from build123d import *

# Parameters (mm, degrees)
SKETCH1_R           = 8.5
SKETCH1_R_2         = 4.5
BOSS_EXTRUDE1_DEPTH = 2.5
SKETCH2_R           = 8
SKETCH2_R_2         = 5
CUT_EXTRUDE1_DEPTH  = 0.1


with BuildPart() as part:
    # Sketch1 → Boss-Extrude1 (new body, symmetric)
    with BuildSketch(Plane(origin=(0, 0, 0), x_dir=(1, 0, 0), z_dir=(0, 1, 0))):
        Circle(SKETCH1_R)
        Circle(SKETCH1_R_2, mode=Mode.SUBTRACT)
    extrude(amount=BOSS_EXTRUDE1_DEPTH, both=True)

    # Sketch2 → Cut-Extrude1 (cut)
    with BuildSketch(Plane(origin=(0, 2.5, 0), x_dir=(1, 0, 0), z_dir=(0, 1, 0))):
        Circle(SKETCH2_R)
        Circle(SKETCH2_R_2, mode=Mode.SUBTRACT)
    cut_extrude1 = extrude(amount=-CUT_EXTRUDE1_DEPTH, mode=Mode.SUBTRACT)

    # Mirror1: Cut-Extrude1 across plane
    add(cut_extrude1.mirror(Plane.ZX), mode=Mode.SUBTRACT)


solid = part.part
Could you check a few things on this model? Use its own coordinates, in mm. A direction names the side the tool comes from. Coordinates: 2 decimals unless noted, no trailing zeros. Write each loop counter-clockwise with the first axis right and the second up, starting at its lowest first coordinate (ties: lowest second). Pieces come first, ordered by that corner, then holes. Notation, with made-up numbers: (38, 45.5) - (81, 45.5) arc R14 cw to (81, 68.5) - close; hole circle Ø3 at (-17.75, -38.5). An arc over 180 degrees is marked (long way). Write item = value, one per line.
1) Suppose I cut it at B-B on z = 0. Please give me the cut outline in (x, y), plus the area to 3 significant figures.
Result set:
outline = (-8.5, -2.5) - (-8, -2.5) - (-8, -2.4) - (-5, -2.4) - (-5, -2.5) - (-4.5, -2.5) - (-4.5, 2.5) - (-5, 2.5) - (-5, 2.4) - (-8, 2.4) - (-8, 2.5) - (-8.5, 2.5) - close; (4.5, -2.5) - (5, -2.5) - (5, -2.4) - (8, -2.4) - (8, -2.5) - (8.5, -2.5) - (8.5, 2.5) - (8, 2.5) - (8, 2.4) - (5, 2.4) - (5, 2.5) - (4.5, 2.5) - close
area = 38.8 mm2
2) Suppose I cut it at A-A on x = 0. Please give me the cut outline in (y, z), plus the area to 3 significant figures.
Result set:
outline = (-2.5, -8.5) - (2.5, -8.5) - (2.5, -8) - (2.4, -8) - (2.4, -5) - (2.5, -5) - (2.5, -4.5) - (-2.5, -4.5) - (-2.5, -5) - (-2.4, -5) - (-2.4, -8) - (-2.5, -8) - close; (-2.5, 4.5) - (2.5, 4.5) - (2.5, 5) - (2.4, 5) - (2.4, 8) - (2.5, 8) - (2.5, 8.5) - (-2.5, 8.5) - (-2.5, 8) - (-2.4, 8) - (-2.4, 5) - (-2.5, 5) - close
area = 38.8 mm2
3) We'd pull the mould along Z, two halves only. Please class faces 1 (the cylindrical face through (4.57, 0.035, -7.167)), 2 (the cylindrical face through (-0.59, -0.04, -4.46)): +Z half, -Z half, draft (parallel to the pull), parting line (faces both ways), or undercut.
Result set:
face_1 = parting line
face_2 = undercut
4) Suppose I cut it at C-C on y = -1.9. Please give me the cut outline in (x, z).
Result set:
outline = circle Ø17 at (0, 0); hole circle Ø9 at (0, 0)
5) For faces 3 (the flat face through (5.2, -2.4, -0.1)), 4 (the flat face through (5.2, 2.4, -0.1)), which set-ups out of +Z, -Z, +X, -X, +Y, -Y let a thin tool reach every point of the face, with its end or its side?
Result set:
face_3 = -Y
face_4 = +Y
6) Will this pin go through, and if not, where does the flat tip stop? pin 1 Ø1.5 at (y, z) = (0.5, 1) entering from -X.
Result set:
pin_1 = -8.5
7) Suppose I cut it at D-D on z = 5.25. Please give me the cut outline in (x, y).
Result set:
outline = (-6.68, -2.5) - (-6.04, -2.5) - (-6.04, -2.4) - (6.04, -2.4) - (6.04, -2.5) - (6.68, -2.5) - (6.68, 2.5) - (6.04, 2.5) - (6.04, 2.4) - (-6.04, 2.4) - (-6.04, 2.5) - (-6.68, 2.5) - close
8) Please list where these lines run through material, in increasing order: line 1 (X direction, y = 2.45, z = 0); line 2 (Z direction, x = 0, y = 0.6); line 3 (Y direction, x = -5, z = 2). Write a range as [from, to].
Result set:
line_1 = [-8.5, -8], [-5, -4.5], [4.5, 5], [8, 8.5]
line_2 = [-8.5, -4.5], [4.5, 8.5]
line_3 = [-2.4, 2.4]
